Work out the finished part from the listing and answer in its coordinate system (mm). Round coordinates to 2 decimals unless told otherwise and drop trailing zeros. Order: outer loops, then holes, each group sorted by start corner. A loop starts at its lowest first (then second) coordinate and runs counter-clockwise, first axis right, second up. Notation, with made-up numbers: (38.5, 63) -> (42.5, 63) arc R20 cw to (42.5, 77) -> close; hole circle Ø10 at (-38, 65). An arc over 180 degrees is marked (long way). Use a Markdown table: item, result. Add a question column.
Item 1: A cutting plane is placed at C-C, the plane z = 23.5. Determine the outline of the cut face in (x, y) (1 decimal), plus the area to 3 significant figures.
Item 2: Find the intervals of material crossed by L1, parallel to Y at x = 10, z = 9; L2, parallel to X at y = -56, z = 54; L3, parallel to X at y = -63.5, z = 41.5, in increasing order. Write a range as [from, to].
Item 3: Flat-ended cylindrical pins translate along their axes: P1, Ø1, axis at y = -58, z = 65.5, coming from the -X side; P2, Ø6, axis at y = -56.5, z = 64, coming from the -X side; P3, Ø5, axis at y = -57.5, z = 23.5, coming from the +X side. Find the tip coordinate at first contact, or state that the pin passes through.
Item 4: A cutting plane is placed at A-A, the plane z = 69.5. Determine the outline of the cut face in (x, y) (1 decimal), plus the area to 3 significant figures.
Item 5: A cutting plane is placed at B-B, the plane z = 55.5. Determine the outline of the cut face in (x, y) (1 decimal), plus the area to 3 significant figures.
from build123d import *

# Parameters (mm, degrees)
F2_ANGLE = 30
F7_DEPTH = 12.7
F8_R     = 1.27


with BuildPart() as f2:
    # F0 (on Right) → F2 (revolve)
    with BuildSketch(Plane.YZ):
        Polygon((-63.5, 0), (0, 0), (0, 25.4), (0, 50.8), (0, 76.2), (-73.025, 76.2), (-69.85, 50.8), (-66.675, 25.4), align=None)
    revolve(axis=Axis((0, 0, 0), (0, 0, 1)), revolution_arc=F2_ANGLE)

    # F3 (on Right) → F5 (revolve, cut)
    with BuildSketch(Plane.YZ):
        Polygon((-57.15, 0), (0, 0), (0, 25.4), (0, 50.8), (0, 76.2), (-66.675, 76.2), align=None)
    revolve(axis=Axis((0, 0, 0), (0, 0, 1)), mode=Mode.SUBTRACT)

    # F6 (on face) → F7 (cut)
    with BuildSketch(Plane.XY.offset(76.2)):
        with BuildLine():
            Line((24.9760209664, -68.6210536329), (0, 0))
            Line((0, 0), (12.6806581741, -71.9155861637))
            ThreePointArc((12.6806581741, -71.9155861637), (20.6260152492, -76.9773368677), (24.9760209664, -68.6210536329))
        make_face()
    extrude(amount=-F7_DEPTH, mode=Mode.SUBTRACT)

    # F8
    f8_edges = [f2.edges().sort_by_distance(p)[0] for p in [
        (12.129325, -68.788822, 76.2),
        (23.890107, -65.63753, 76.2),
        (34.925, -60.491874, 76.2),
        (30.1625, -52.242982, 0),
        (0, -60.325, 0),
        (0, -69.85, 76.2),
        (11.853659, -67.225439, 63.5),
        (23.34715, -64.145768, 63.5),
    ]]
    fillet(f8_edges, radius=F8_R)


solid = f2.part
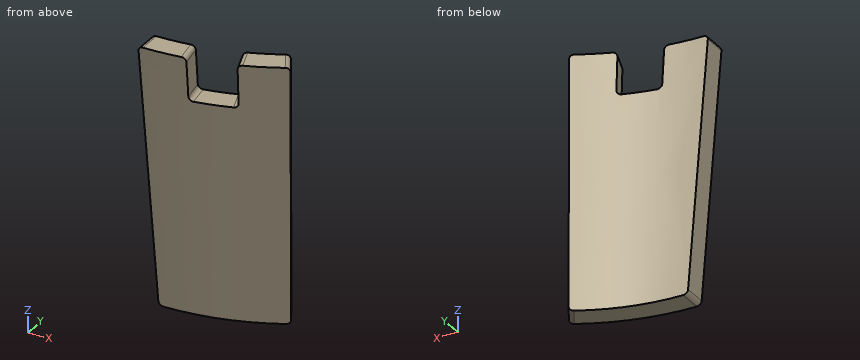
Reported:
| question | item | result |
|---|---|---|
| 1 | outline | (0, -66.4) arc R66.4 ccw to (33.2, -57.5) -> (30, -52) arc R60.1 cw to (0, -60.1) -> close |
| 1 | area | 210 mm² |
| 2 | L1 | [-63.85, -57.41] |
| 2 | L2 | [30.78, 32.33] |
| 2 | L3 | [0, 26.19] |
| 3 | P1 | x = 29.09 |
| 3 | P2 | x = 26.48 |
| 3 | P3 | x = 33.37 |
| 4 | outline | (0, -72.2) arc R72.2 ccw to (12.5, -71.1) -> (11.4, -64.8) arc R65.8 cw to (0, -65.8) -> close; (22.5, -61.9) -> (24.7, -67.8) arc R72.2 ccw to (36.1, -62.5) -> (32.9, -57) arc R65.8 cw to start |
| 4 | area | 153 mm² |
| 5 | outline | (0, -70.4) arc R70.4 ccw to (35.2, -61) -> (32, -55.5) arc R64.1 cw to (0, -64.1) -> close |
| 5 | area | 224 mm² |
